Can you work these out from the model? Positions are in its coordinate system, mm. A direction names the side the tool comes from. Round coordinates to 2 decimals unless told otherwise and drop trailing zeros. Write each loop counter-clockwise with the first axis right and the second up, starting at its lowest first coordinate (ties: lowest second). Pieces come first, ordered by that corner, then holes.
Q1. We'd pull the mould along X, two halves only. Please class faces 1 (the flat face through (-1, 2, -65)), 2 (the flat face through (50, 2, -60)), 3 (the cylindrical face through (45.734, 1.521, 56.357)): +X half, -X half, draft (parallel to the pull), parting line (faces both ways), or undercut.
Q2. For faces 4 (the flat face through (39, 2, -55)), 5 (the flat face through (-27.5, 2, -2)), 6 (the cylindrical face through (43.226, 1.521, -59.077)), 7 (the flat face through (-50, 2, -60)), 8 (the flat face through (-1, 2, 59.51)), which set-ups out of +Z, -Z, +X, -X, +Y, -Y let a thin tool reach every point of the face, with its end or its side?
Q3. I'm going to push flat-ended pins straight in: pin 1 Ø1.5 at (y, z) = (1, -25.5) entering from -X; pin 2 Ø5 at (x, z) = (-47.5, 54.51) entering from -Y. Where does each tip first touch, or does it pass through?
Q4. If we section it at C-C (z = 54.51): Please give me the cut outline in (x, y), plus the area to 3 significant figures.
Q5. If we section it at A-A (z = -29.2): Please give me the cut outline in (x, y), plus the area to 3 significant figures.
Q6. If we section it at D-D (y = 1.9): Please give me the cut outline in (x, z).
Q7. If we section it at B-B (x = -8.9): Please give me the cut outline in (y, z), plus the area to 3 significant figures.
Q8. Please list where these lines run through material, in increasing order: line 1 along X through (y, z) = (1.4, -60); line 2 along Z through (x, y) = (-37, 2.85); line 3 along X through (y, z) = (1.45, 54.51).
from build123d import *

# Parameters (mm, degrees)
CROQUIS1_R              = 75
SALIENTE_EXTRUIR1_DEPTH = 3
CROQUIS5_W              = 55
CROQUIS5_H              = 104.51
CORTAR_EXTRUIR10_DEPTH  = 107.108435103
CROQUIS10_W             = 100
CROQUIS10_H             = 10
CROQUIS10_R             = 2
SALIENTE_EXTRUIR2_DEPTH = 3
CROQUIS12_W             = 104
CROQUIS12_H             = 10
CROQUIS12_R             = 2
SALIENTE_EXTRUIR3_DEPTH = 3
CROQUIS13_R             = 1.5
CORTAR_EXTRUIR11_DEPTH  = 84.294657692


with BuildPart() as part:
    # Croquis1 → Saliente-Extruir1 (new body)
    with BuildSketch(Plane(origin=(0, 0, 0), x_dir=(1, 0, 0), z_dir=(0, 1, 0))):
        with Locations(Location((0, 0, 0), (0, 0, 270))):
            Circle(CROQUIS1_R)
    extrude(amount=SALIENTE_EXTRUIR1_DEPTH)

    # Croquis5 → Cortar-Extruir10 (cut, through all)
    with BuildSketch(Plane(origin=(0, 3, 0), x_dir=(1, 0, 0), z_dir=(0, 1, 0))):
        Polygon((53, 55), (53, 77), (-53, 77), (-53, 55), (-77.5, 55), (-77.5, -70), (-27.5, -70), (-27.5, -78), (27.5, -78), (27.5, -70), (75, -70), (75, 55), align=None)
        with Locations((0, 2.745)):
            Rectangle(CROQUIS5_W, CROQUIS5_H, mode=Mode.SUBTRACT)
    extrude(amount=-CORTAR_EXTRUIR10_DEPTH, mode=Mode.SUBTRACT)

    # Croquis10 → Saliente-Extruir2 (add)
    with BuildSketch(Plane(origin=(0, 3, 0), x_dir=(1, 0, 0), z_dir=(0, 1, 0))):
        with Locations((0, 60)):
            Rectangle(CROQUIS10_W, CROQUIS10_H)
        with Locations(Location((-45, 60, 0), (0, 0, 270))):
            Circle(CROQUIS10_R, mode=Mode.SUBTRACT)
        with Locations(Location((45, 60, 0), (0, 0, 270))):
            Circle(CROQUIS10_R, mode=Mode.SUBTRACT)
    extrude(amount=-SALIENTE_EXTRUIR2_DEPTH)

    # Croquis12 → Saliente-Extruir3 (add)
    with BuildSketch(Plane(origin=(0, 3, 0), x_dir=(1, 0, 0), z_dir=(0, 1, 0))):
        with Locations((0, -54.51)):
            Rectangle(CROQUIS12_W, CROQUIS12_H)
        with Locations(Location((-47.5, -54.51, 0), (0, 0, 270))):
            Circle(CROQUIS12_R, mode=Mode.SUBTRACT)
        with Locations(Location((46.5, -54.51, 0), (0, 0, 270))):
            Circle(CROQUIS12_R, mode=Mode.SUBTRACT)
    extrude(amount=-SALIENTE_EXTRUIR3_DEPTH)

    # Croquis13 → Cortar-Extruir11 (cut, through all)
    with BuildSketch(Plane(origin=(0, 3, 0), x_dir=(1, 0, 0), z_dir=(0, 1, 0))):
        with Locations(Location((-8.9, 29.2, 0), (0, 0, 270))):
            Circle(CROQUIS13_R)
    extrude(amount=-CORTAR_EXTRUIR11_DEPTH, mode=Mode.SUBTRACT)


solid = part.part
A:
1. face 1: draft
1. face 2: +X half
1. face 3: undercut
2. face 4: +X, +Y, -Y
2. face 5: -X, +Y, -Y
2. face 6: +Y, -Y
2. face 7: -Z, -X, +Y, -Y
2. face 8: +Z, +X, -X, +Y, -Y
3. pin 1: stops at x = -27.5
3. pin 2: stops at y = 0
4. outline: (-52, 0) - (-49.5, 0) - (-49.5, 3) - (-52, 3) - close; (-45.5, 0) - (44.5, 0) - (44.5, 3) - (-45.5, 3) - close; (48.5, 0) - (52, 0) - (52, 3) - (48.5, 3) - close
4. area: 288 mm2
5. outline: (-27.5, 0) - (-10.4, 0) - (-10.4, 3) - (-27.5, 3) - close; (-7.4, 0) - (27.5, 0) - (27.5, 3) - (-7.4, 3) - close
5. area: 156 mm2
6. outline: (-52, 49.51) - (-27.5, 49.51) - (-27.5, -55) - (-50, -55) - (-50, -65) - (50, -65) - (50, -55) - (27.5, -55) - (27.5, 49.51) - (52, 49.51) - (52, 59.51) - (-52, 59.51) - close; hole circle Ø4 at (-47.5, 54.51); hole circle Ø4 at (-45, -60); hole circle Ø3 at (-8.9, -29.2); hole circle Ø4 at (45, -60); hole circle Ø4 at (46.5, 54.51)
7. outline: (0, -65) - (3, -65) - (3, -30.7) - (0, -30.7) - close; (0, -27.7) - (3, -27.7) - (3, 59.51) - (0, 59.51) - close
7. area: 365 mm2
8. line 1: x = -50 to -47, -43 to 43, 47 to 50
8. line 2: z = -65 to -55, 49.51 to 59.51
8. line 3: x = -52 to -49.5, -45.5 to 44.5, 48.5 to 52
